Geometry: see drawing. Coordinates: mm, zero at the bounding-box minimum. Give positions to 0.01 mm unless a question says otherwise; leave off trailing zeros. Write each loop counter-clockwise with the first axis right and the second up, starting at its lowest first coordinate (ties: lowest second). Pieces come first, ordered by that corner, then holes. Notation, with made-up numbers: M 38,75 L 42,75 A15 ccw 42,103 Z; hole C 79,-29.75 d7. An arc over 180 degrees is marked long. Use a Markdown table: item, result. Add a question column.
1) Section B-B on z = 1.25. Return the cut outline in (x, y), then the cut area to 3 significant figures.
2) Section C-C on y = 4. Return the cut outline in (x, z).
3) Pin query (flat end, axial travel): pin 1 (1.2 mm diameter, centred on x = 32.5, y = 5, fed in from -Z); pin 2 (1.8 mm diameter, centred on x = 32.297, y = 4, fed in from -Z). Return the tip coordinate at first contact, or that it passes through.
4) Line query: line 1 (X direction, y = 4.25, z = 0.55) (1 decimal); line 2 (Y direction, x = 4, z = 2.1); line 3 (X direction, y = 3, z = 1.15) (1 decimal). Output: solid intervals per line, ascending.
5) Section A-A on x = 4. Return the cut outline in (y, z).
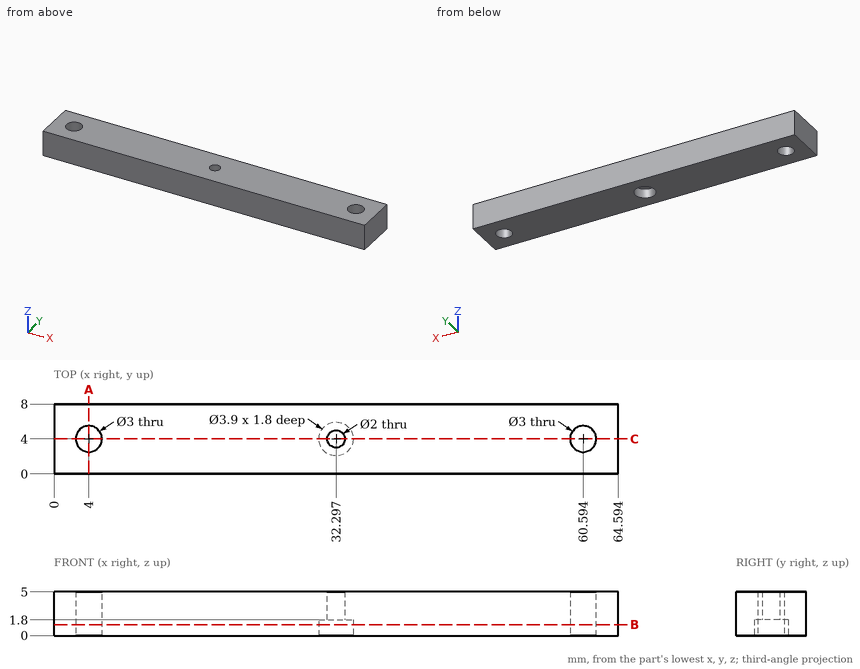
Found:
| question | item | result |
|---|---|---|
| 1 | outline | M 0,0 L 64.59,0 L 64.59,8 L 0,8 Z; hole C 4,4 d3; hole C 32.3,4 d3.9; hole C 60.59,4 d3 |
| 1 | area | 491 mm² |
| 2 | outline | M 0,0 L 2.5,0 L 2.5,5 L 0,5 Z; M 5.5,0 L 30.35,0 L 30.35,1.8 L 31.3,1.8 L 31.3,5 L 5.5,5 Z; M 33.3,1.8 L 34.25,1.8 L 34.25,0 L 59.09,0 L 59.09,5 L 33.3,5 Z; M 62.09,0 L 64.59,0 L 64.59,5 L 62.09,5 Z |
| 3 | pin 1 | z = 1.8 |
| 3 | pin 2 | through |
| 4 | line 1 | 0 to 2.5, 5.5 to 30.4, 34.2 to 59.1, 62.1 to 64.6 |
| 4 | line 2 | 0 to 2.5, 5.5 to 8 |
| 4 | line 3 | 0 to 2.9, 5.1 to 30.6, 34 to 59.5, 61.7 to 64.6 |
| 5 | outline | M 0,0 L 2.5,0 L 2.5,5 L 0,5 Z; M 5.5,0 L 8,0 L 8,5 L 5.5,5 Z |
